Autodesk Inventor part; units mm, degrees
ref_plane "YZ Plane" through (0, 0, 0) normal (1, 0, 0) x (0, 1, 0)
ref_plane "XZ Plane" through (0, 0, 0) normal (0, 1, 0) x (-1, 0, 0)
ref_plane "XY Plane" through (0, 0, 0) normal (0, 0, 1) x (1, 0, 0)
sketch "スケッチ1" plane through (0, 0, 0) normal (0, 0, 1) x (1, 0, 0)
  line L0 (8.75, 11.25) -> (12.25, 11.25)
  line L1 (14.25, 9.25) -> (14.25, -33.25)
  line L2 (12.25, -35.25) -> (-12.25, -35.25)
  line L3 (-14.25, -33.25) -> (-14.25, -29.75)
  line L4 (-12.25, 11.25) -> (-14.25, 9.25)
  line L5 (12.25, 11.25) -> (14.25, 9.25)
  line L6 (14.25, -33.25) -> (12.25, -35.25)
  line L7 (-12.25, -35.25) -> (-14.25, -33.25)
  line L8 (0, 0) -> (-26.5626, 0) construction
  line L9 (0, 0) -> (0, 27.9433) construction
  line L10 (-11, 8) -> (11, 8) construction
  line L11 (11, 8) -> (11, -32) construction
  line L12 (11, -32) -> (-11, -32) construction
  line L13 (-11, -32) -> (-11, 8) construction
  line L14 (-13.15, -28.5) -> (-13.15, 4.5) construction
  line L15 (-7.5, 10.15) -> (7.5, 10.15) construction
  line L16 (13.15, 4.5) -> (13.15, -28.5)
  line L17 (7.5, -34.15) -> (-7.5, -34.15)
  line L18 (8.5, 8) -> (8.5, 11)
  line L19 (11, 5.5) -> (12.15, 5.5)
  arc A0 (8.5, 8) -> (11, 5.5) centre (11, 8) ccw
  line L20 (12.15, -29.5) -> (11, -29.5)
  line L21 (8.5, -32) -> (8.5, -33.15)
  arc A1 (11, -29.5) -> (8.5, -32) centre (11, -32) ccw
  line L22 (-8.5, 8) -> (-8.5, 9.15) construction
  line L23 (-11, 5.5) -> (-12.15, 5.5) construction
  arc A2 (-11, 5.5) -> (-8.5, 8) centre (-11, 8) ccw construction
  line L24 (-14, -29.5) -> (-11, -29.5)
  line L25 (-8.5, -32) -> (-8.5, -33.15)
  arc A3 (-8.5, -32) -> (-11, -29.5) centre (-11, -32) ccw
  arc A4 (8.5, 9.15) -> (7.5, 10.15) centre (7.5, 9.15) ccw construction
  arc A5 (13.15, 4.5) -> (12.15, 5.5) centre (12.15, 4.5) ccw
  arc A6 (12.15, -29.5) -> (13.15, -28.5) centre (12.15, -28.5) ccw
  arc A7 (7.5, -34.15) -> (8.5, -33.15) centre (7.5, -33.15) ccw
  arc A8 (-8.5, -33.15) -> (-7.5, -34.15) centre (-7.5, -33.15) ccw
  arc A9 (-13.15, -28.5) -> (-12.15, -29.5) centre (-12.15, -28.5) ccw construction
  arc A10 (-12.15, 5.5) -> (-13.15, 4.5) centre (-12.15, 4.5) ccw construction
  arc A11 (-7.5, 10.15) -> (-8.5, 9.15) centre (-7.5, 9.15) ccw construction
  line L26 (8.75, 11.25) -> (8.5, 11)
  line L27 (-14, -29.5) -> (-14.25, -29.75)
  point P0 (-14.25, 11.25)
  point P1 (14.25, -35.25)
  point P2 (14.25, 11.25)
  point P3 (-14.25, -35.25)
  point P4 (8.5, 10.15)
  point P5 (13.15, 5.5)
  point P6 (13.15, -29.5)
  point P7 (8.5, -34.15)
  point P8 (-8.5, 10.15)
  point P9 (-13.15, 5.5)
  point P10 (-13.15, -29.5)
  point P11 (-8.5, -34.15)
  point P12 (8.5, 11.25)
  point P13 (-14.25, -29.5)
  dimension "d0" = 2
  dimension "d1" = 2
  dimension "d2" = 2
  dimension "d3" = 2
  dimension "d4" = 2
  dimension "d5" = 2
  dimension "d6" = 2
  dimension "d7" = 2
  dimension "d8" = 28.5
  dimension "d9" = 11.25
  dimension "d10" = 46.5
  dimension "d11" = 8
  dimension "d12" = 22
  dimension "d13" = 40
  dimension "d14" = 1.1
  dimension "d15" = 2.5
  dimension "d16" = 2.5
  dimension "d17" = 1.1
  dimension "d18" = 1.1
  dimension "d19" = 1
  dimension "d35" = 0.25
  dimension "d36" = 0.25
  dimension "d37" = 0.25
  dimension "d38" = 0.25
extrude "押し出し1" add sketch "スケッチ1" along normal blind 3.1
hole "穴1" at (-11, 8, 0) at (11, 8, 0) at (11, -32, 0) at (-11, -32, 0) direction (0, 0, 1) diameter 2.5 end through all
sketch "スケッチ3" plane through (0, 0, 0) normal (0, 0, -1) x (-1, 0, 0)
  line L0 (-8.75, 11.25) -> (-12.25, 11.25) construction
  line L1 (14.25, -33.25) -> (14.25, -29.75) construction
  line L2 (12.25, -35.25) -> (14.25, -33.25) construction
  line L3 (-12.25, -35.25) -> (12.25, -35.25) construction
  line L4 (-14.25, -33.25) -> (-12.25, -35.25) construction
  line L5 (-14.25, 9.25) -> (-14.25, -33.25) construction
  line L6 (-12.25, 11.25) -> (-14.25, 9.25) construction
  line L7 (-8.5, 10.625) -> (-11.087, 10.625)
  line L8 (-11.9911, 10.625) -> (-13.625, 8.9911) construction
  line L9 (-13.625, 8.087) -> (-13.625, -32.087)
  line L10 (-13.625, -32.9911) -> (-11.9911, -34.625) construction
  line L11 (-11.087, -34.625) -> (11.087, -34.625)
  line L12 (11.9911, -34.625) -> (13.625, -32.9911) construction
  line L13 (13.625, -32.087) -> (13.625, -29.5)
  line L14 (-13.1857, -33.1476) -> (-12.1476, -34.1857)
  line L15 (12.1476, -34.1857) -> (13.1857, -33.1476)
  line L16 (-13.1857, 9.1476) -> (-12.1476, 10.1857)
  arc A0 (-13.1857, 9.1476) -> (-13.625, 8.087) centre (-12.125, 8.087) ccw
  arc A1 (-11.087, 10.625) -> (-12.1476, 10.1857) centre (-11.087, 9.125) ccw
  arc A2 (13.1857, -33.1476) -> (13.625, -32.087) centre (12.125, -32.087) ccw
  arc A3 (11.087, -34.625) -> (12.1476, -34.1857) centre (11.087, -33.125) ccw
  arc A4 (-12.1476, -34.1857) -> (-11.087, -34.625) centre (-11.087, -33.125) ccw
  arc A5 (-13.625, -32.087) -> (-13.1857, -33.1476) centre (-12.125, -32.087) ccw
  arc A6 (-12.15, 5.5) -> (-13.15, 4.5) centre (-12.15, 4.5) ccw
  line L17 (-12.15, 5.5) -> (-11, 5.5)
  arc A7 (-11, 5.5) -> (-8.5, 8) centre (-11, 8) ccw
  line L18 (-8.5, 8) -> (-8.5, 11) construction
  line L19 (14, -29.5) -> (11, -29.5) construction
  arc A8 (11, -29.5) -> (8.5, -32) centre (11, -32) ccw
  line L20 (8.5, -32) -> (8.5, -33.15)
  arc A9 (7.5, -34.15) -> (8.5, -33.15) centre (7.5, -33.15) ccw
  circle A10 centre (11, -32) radius 1.25
  line L21 (7.5, -34.15) -> (-7.5, -34.15)
  arc A11 (-8.5, -33.15) -> (-7.5, -34.15) centre (-7.5, -33.15) ccw
  line L22 (-8.5, -33.15) -> (-8.5, -32)
  arc A12 (-8.5, -32) -> (-11, -29.5) centre (-11, -32) ccw
  line L23 (-11, -29.5) -> (-12.15, -29.5)
  arc A13 (-13.15, -28.5) -> (-12.15, -29.5) centre (-12.15, -28.5) ccw
  circle A14 centre (-11, -32) radius 1.25
  line L24 (-13.15, -28.5) -> (-13.15, 4.5)
  circle A15 centre (-11, 8) radius 1.25
  line L25 (11, -29.5) -> (13.625, -29.5)
  line L26 (-8.5, 8) -> (-8.5, 10.625)
  point P0 (0, 0)
  dimension "d30" = 0.625
  dimension "d31" = 1.5
  dimension "d32" = 0.2
  dimension "d39" = 0.625
  dimension "d40" = 0.625
  dimension "d41" = 0.2
extrude "押し出し2" add sketch "スケッチ3" along normal blind 0.75
properties part number "COXA_YAW_ROLL_ADPT_SPACER"
Input: part model. Units: mm. Frame: model coordinates. A direction names the side the tool comes from. Round coordinates to 2 decimals unless told otherwise and drop trailing zeros. Order: outer loops, then holes, each group sorted by start corner. A loop starts at its lowest first (then second) coordinate and runs counter-clockwise, first axis right, second up. Notation, with made-up numbers: (-13, -32.75) - (16, -32.75) arc R34 cw to (16, -2.75) - close; hole circle Ø2 at (55.5, -30). An arc over 180 degrees is marked (long way). Answer as a JSON object with one key per item and string values. Group by question number.
(1) Pin query (flat end, axial travel): P1, Ø2, axis at x = -11, y = -32, coming from the -Z side; P2, Ø0.8, axis at x = 0, z = -0.5, coming from the -Y side (3 decimals); P3, Ø1.5, axis at y = 10, z = 1.5, coming from the -X side; P4, Ø2, axis at x = -6, z = -0.5, coming from the +Y side. Return the tip coordinate at first contact, or that it passes through.
(2) Draft query along Y for faces 1 (the face through (9.9, -31.41, 1.2)), 2 (the face through (-9.213, -30.252, 1.202)), 3 (the face through (-14.25, -32, 2)). Return one class per face: released by +Y, released by -Y, zero draft, split by the parting line, or undercut.
(3) Cut plane A-A (z = 1). Return loops of the section in (x, y).
(4) Material intervals for probe 1 along Y at (x, z) = (11, 0.4); probe 2 along X at (y, z) = (8, 0.1); probe 3 along X at (y, z) = (-32, 1.7), sorted ascending. Write a range as from..to.
(5) Cut plane B-B (y = -17.5). Return loops of the section in (x, z) (3 decimals).
(6) Cut plane C-C (x = -5.75). Return loops of the section in (y, z) (3 decimals), then the cut area to 3 significant figures.
(7) Reachability of faces 4 (the face through (-8.215, -33.849, 1.202)), 5 (the face through (12.674, -33.659, -0.37)), 6 (the face through (12.849, -29.215, 1.202)), 7 (the face through (-12.659, -33.674, -0.37)) from +Z, -Z, +X, -X, +Y, -Y: full face, straight path, thin tool, end or side. Return the list, or none.
Here are the results:
{
 "1": {"P1": "passes through", "P2": "stops at y = -34.625", "P3": "stops at x = 8.5", "P4": "stops at y = -34.15"},
 "2": {"face 1": "undercut", "face 2": "released by +Y", "face 3": "zero draft"},
 "3": {"outline": "(-14.25, -33.25) - (-12.25, -35.25) - (12.25, -35.25) - (14.25, -33.25) - (14.25, 9.25) - (12.25, 11.25) - (8.75, 11.25) - (8.5, 11) - (8.5, 8) arc R2.5 ccw to (11, 5.5) - (12.15, 5.5) arc R1 cw to (13.15, 4.5) - (13.15, -28.5) arc R1 cw to (12.15, -29.5) - (11, -29.5) arc R2.5 ccw to (8.5, -32) - (8.5, -33.15) arc R1 cw to (7.5, -34.15) - (-7.5, -34.15) arc R1 cw to (-8.5, -33.15) - (-8.5, -32) arc R2.5 ccw to (-11, -29.5) - (-14, -29.5) - (-14.25, -29.75) - close; hole circle Ø2.5 at (-11, -32); hole circle Ø2.5 at (11, -32); hole circle Ø2.5 at (11, 8)"},
 "4": {"probe 1": "y = -35.25..-33.25, -30.75..-29.5, 5.5..6.75, 9.25..11.25", "probe 2": "x = 8.5..9.75, 12.25..14.25", "probe 3": "x = -14.25..-12.25, -9.75..-8.5, 8.5..9.75, 12.25..14.25"},
 "5": {"outline": "(13.15, -0.75) - (13.625, -0.75) - (13.625, 0) - (14.25, 0) - (14.25, 3.1) - (13.15, 3.1) - close"},
 "6": {"outline": "(-35.25, 0) - (-34.625, 0) - (-34.625, -0.75) - (-34.15, -0.75) - (-34.15, 3.1) - (-35.25, 3.1) - close", "area": "3.77 mm^2"},
 "7": {"face 4": "+Z, -Z, +Y", "face 5": "-Z, +X, -Y", "face 6": "+Z, -Z, -X", "face 7": "-Z, -X, -Y"}
}
